The listing builds one solid part. Answer for the finished solid, in the listing's coordinates (mm). A direction names the side the tool comes from. Coordinates: 2 decimals unless noted, no trailing zeros. Loops run counter-clockwise (first coordinate to the right, second up) from the corner with the lowest first, then second, coordinate; pieces in that order, holes last. Notation, with made-up numbers: M 13.25,-14 L 64.25,-14 A25 cw 64.25,15 Z; hole C 68.25,35 d6. An arc over 180 degrees is marked long. Answer in a Markdown table with one row per item. Add a question column.
from build123d import *

# Parameters (mm, degrees)
SKETCH_1_W          = 30
SKETCH_1_H          = 16
EXTRUDE_1_DEPTH     = 3
SKETCH_2_W          = 3
SKETCH_2_H          = 16
EXTRUDE_2_DEPTH     = 29
SKETCH_4_W          = 16
SKETCH_4_H          = 3
EXTRUDE_3_DEPTH     = 6
SKETCH_5_W          = 16
SKETCH_5_H          = 3
EXTRUDE_4_DEPTH     = 6
SKETCH_6_R          = 5.5
CUT_EXTRUDE_1_DEPTH = 41.792156109
SKETCH_7_R          = 1.5
CUT_EXTRUDE_2_DEPTH = 37.235341864
FILLET_1_R          = 3


with BuildPart() as part:
    # 草图1 → 凸台-拉伸1 (new body)
    with BuildSketch(Plane(origin=(0, 0, 0), x_dir=(1, 0, 0), z_dir=(0, 1, 0))):
        Rectangle(SKETCH_1_W, SKETCH_1_H)
    extrude(amount=EXTRUDE_1_DEPTH)

    # 草图2 → 凸台-拉伸2 (add)
    with BuildSketch(Plane(origin=(0, 3, 0), x_dir=(1, 0, 0), z_dir=(0, 1, 0))):
        with Locations((7.5, 0)):
            Rectangle(SKETCH_2_W, SKETCH_2_H)
        with Locations((-7.5, 0)):
            Rectangle(SKETCH_2_W, SKETCH_2_H)
    extrude(amount=EXTRUDE_2_DEPTH)

    # 草图4 → 凸台-拉伸3 (add)
    with BuildSketch(Plane.ZY.offset(9)):
        with Locations((0, 30.5)):
            Rectangle(SKETCH_4_W, SKETCH_4_H)
    extrude(amount=EXTRUDE_3_DEPTH)

    # 草图5 → 凸台-拉伸4 (add)
    with BuildSketch(Plane(origin=(9, 0, 0), x_dir=(0, 0, -1), z_dir=(1, 0, 0))):
        with Locations((0, 30.5)):
            Rectangle(SKETCH_5_W, SKETCH_5_H)
    extrude(amount=EXTRUDE_4_DEPTH)

    # 草图6 → 切除-拉伸1 (cut, through all)
    with BuildSketch(Plane(origin=(9, 0, 0), x_dir=(0, 0, -1), z_dir=(1, 0, 0))):
        with Locations((0, 16)):
            Circle(SKETCH_6_R)
    extrude(amount=-CUT_EXTRUDE_1_DEPTH, mode=Mode.SUBTRACT)

    # 草图7 → 切除-拉伸2 (cut, through all)
    with BuildSketch(Plane(origin=(0, 32, 0), x_dir=(1, 0, 0), z_dir=(0, 1, 0))):
        with Locations(Location((12, 5, 0), (0, 0, 270))):
            Circle(SKETCH_7_R)
        with Locations(Location((12, -5, 0), (0, 0, 270))):
            Circle(SKETCH_7_R)
        with Locations(Location((-12, -5, 0), (0, 0, 270))):
            Circle(SKETCH_7_R)
        with Locations(Location((-12, 5, 0), (0, 0, 270))):
            Circle(SKETCH_7_R)
    extrude(amount=-CUT_EXTRUDE_2_DEPTH, mode=Mode.SUBTRACT)

    # 圆角1
    fillet_1_edges = [part.edges().sort_by_distance(p)[0] for p in [
        (-15, 30.5, -8),
        (-15, 30.5, 8),
        (15, 30.5, 8),
        (15, 30.5, -8),
        (15, 1.5, 8),
        (-15, 1.5, 8),
        (-15, 1.5, -8),
        (15, 1.5, -8),
    ]]
    fillet(fillet_1_edges, radius=FILLET_1_R)


solid = part.part
(1) Straight lines are drawn through the part: line 1 (X direction, y = 1.25, z = -5); line 2 (X direction, y = 29.6, z = 5); line 3 (Y direction, x = -9.25, z = 4.5). For each, find the intervals that lie inside material, in ascending order.
(2) A cutting plane is placed at A-A (y = 16). Give the vertices of the cut face in (x, z).
(3) A cutting plane is placed at D-D (x = -6.75). Give the vertices of the cut face in (y, z), plus the area to 3 significant figures.
(4) For faces 4 (the face through (-9, 22, 0)), 5 (the face through (6, 21, 4)), 6 (the face through (9, 22, 0)), determine the directions among +Z, -Z, +X, -X, +Y, -Y from which every point of the face is accessible in a straight line to the end or side of a thin tool.
(5) A cutting plane is placed at C-C (y = 25.5). Give the vertices of the cut face in (x, z), plus the area to 3 significant figures.
(6) A cutting plane is placed at B-B (z = 0). Give the vertices of the cut face in (x, y), plus the area to 3 significant figures.
(7) Each of these flat-tipped pins is pushed along its axis until it touches: pin 1 (8 mm diameter, centred on y = 18, z = 3.5, fed in from -X); pin 2 (1.5 mm diameter, centred on y = 25, z = -1, fed in from +X); pin 3 (3 mm diameter, centred on x = 4, z = -2.5, fed in from +Y). Where does it stop, or does it pass through?
(8) The mould has two halves that part along Z. Classify faces 1 (the face through (-12.575, 30.521, 6.386)), 2 (the face through (6.2, 14.7, 8)), 3 (the face through (10, 32, 0)): released by +Z, released by -Z, zero draft, split by the parting line, or undercut.
Solved:
| question | item | result |
|---|---|---|
| 1 | line 1 | x = -15 to -13.5, -10.5 to 10.5, 13.5 to 15 |
| 1 | line 2 | x = -15 to -13.5, -10.5 to -6, 6 to 10.5, 13.5 to 15 |
| 1 | line 3 | y = 0 to 3, 29 to 32 |
| 2 | outline | M -9,-8 L -6,-8 L -6,-5.5 L -9,-5.5 Z; M -9,5.5 L -6,5.5 L -6,8 L -9,8 Z; M 6,-8 L 9,-8 L 9,-5.5 L 6,-5.5 Z; M 6,5.5 L 9,5.5 L 9,8 L 6,8 Z |
| 3 | outline | M 0,-8 L 32,-8 L 32,8 L 0,8 Z; hole C 16,0 d11 |
| 3 | area | 417 mm² |
| 4 | face 4 | +Z, -Z, -X |
| 4 | face 5 | +Z, -Z, +Y |
| 4 | face 6 | +Z, -Z, +X |
| 5 | outline | M -9,-8 L -6,-8 L -6,8 L -9,8 Z; M 6,-8 L 9,-8 L 9,8 L 6,8 Z |
| 5 | area | 96.0 mm² |
| 6 | outline | M -15,0 L 15,0 L 15,3 L 9,3 L 9,10.5 L 6,10.5 L 6,3 L -6,3 L -6,10.5 L -9,10.5 L -9,3 L -15,3 Z; M -15,29 L -9,29 L -9,21.5 L -6,21.5 L -6,32 L -15,32 Z; M 6,21.5 L 9,21.5 L 9,29 L 15,29 L 15,32 L 6,32 Z |
| 6 | area | 234 mm² |
| 7 | pin 1 | stops at x = -9 |
| 7 | pin 2 | stops at x = 9 |
| 7 | pin 3 | stops at y = 3 |
| 8 | face 1 | undercut |
| 8 | face 2 | released by +Z |
| 8 | face 3 | zero draft |
